Part model, mm, in its own coordinate system. A direction names the side the tool comes from. Round coordinates to 2 decimals unless told otherwise and drop trailing zeros. Loops run counter-clockwise (first coordinate to the right, second up) from the corner with the lowest first, then second, coordinate; pieces in that order, holes last. Notation, with made-up numbers: (33.25, 74) -> (59.25, 74) arc R15 cw to (59.25, 103) -> close; hole circle Ø10 at (86.25, 63.25). An arc over 180 degrees is marked (long way). Use a Markdown table: item, result. Add a question column.
Item 1: Cut at C-C, the plane y = 12. State how many separate pieces and enclosed holes the cut face has, plus the area to 3 significant figures.
Item 2: Which spindle directions (+Z, -Z, +X, -X, +Y, -Y) get a long thin tool onto all of the face, cutting with end or side? Do faces 1 (the face through (23, 6.35, 0)), 2 (the face through (30.8, 12.5, 25.1)), 3 (the face through (27.111, 18.942, -25.094)). Say none if no direction does.
Item 3: Two-plate mould, pull along X, no slides. Class faces 4 (the face through (-22.953, 39.572, 25.094)), 5 (the face through (5, 28, -25.4)), 6 (the face through (6.854, 38.289, -0.341)), 7 (the face through (-11, 6.35, 0)): pulls with the +X half, pulls with the -X half, needs draft (parallel to the pull), parting line crosses it, or undercut.
Item 4: Flat gauge pins, fed straight in: pin 1 (12 mm diameter, centred on x = -18.5, z = -2, fed in from +Y); pin 2 (3 mm diameter, centred on y = 31, z = -18, fed in from -X); pin 3 (12 mm diameter, centred on y = 14, z = -10, fed in from +X). Where does each tip first touch, or does it go through?
Item 5: Probe line 1 (X direction, y = 9.5, z = -14); line 2 (X direction, y = 11.5, z = -13); line 3 (Y direction, x = 17, z = -20). List the from-to ranges inside material, lowest first. Write a range as [from, to].
Item 6: Cut at B-B, the plane x = 19. List the corners of the cut face in (y, z), plus the area to 3 significant figures.
Autodesk Inventor part; units mm, degrees
ref_plane "YZ Plane" through (0, 0, 0) normal (1, 0, 0) x (0, 1, 0)
ref_plane "XZ Plane" through (0, 0, 0) normal (0, 1, 0) x (-1, 0, 0)
ref_plane "XY Plane" through (0, 0, 0) normal (0, 0, 1) x (1, 0, 0)
sketch "Sketch1" plane through (0, 0, 0) normal (0, 1, 0) x (-1, 0, 0)
  line L0 (-38.1, -25.4) -> (38.1, -25.4)
  line L1 (38.1, -25.4) -> (38.1, 25.4)
  line L2 (38.1, 25.4) -> (-38.1, 25.4)
  line L3 (-38.1, 25.4) -> (-38.1, -25.4)
  line L4 (-38.1, -25.4) -> (38.1, 25.4) construction
  line L5 (38.1, -25.4) -> (-38.1, 25.4) construction
  point P0 (0, 0)
  dimension "d0" = 76.2
  dimension "d1" = 50.8
extrude "Extrusion1" add sketch "Sketch1" along normal blind 6.35
sketch "Sketch2" plane through (38.1, 0, -25.4) normal (0, 0, -1) x (-1, 0, 0)
  line L0 (76.2, 6.35) -> (0, 6.35)
  line L1 (0, 6.35) -> (21.59, 6.35)
  line L2 (21.59, 6.35) -> (43.642, 79.2894)
  line L3 (76.2, 0) -> (76.2, 6.35)
  line L4 (43.642, 79.2894) -> (76.2, 6.35)
  line L5 (76.2, 6.35) -> (69.85, 6.35)
  line L6 (69.85, 6.35) -> (44.8636, 62.3267)
  line L7 (21.59, 6.35) -> (27.94, 6.35) construction
  line L8 (27.94, 6.35) -> (44.8636, 62.3267)
  line L9 (0, 6.35) -> (76.2, 6.35)
  line L10 (10.1092, 9.821) -> (9.0598, 6.35)
  line L11 (9.0598, 6.35) -> (5.2498, 6.35)
  line L12 (5.2498, 6.35) -> (9.0598, 19.7904)
  line L13 (9.0598, 19.7904) -> (12.64, 18.7755)
  line L14 (12.64, 18.7755) -> (9.9878, 9.4194)
  point P0 (38.1, 0)
  point P1 (5.2498, 6.35)
  point P2 (9.0598, 6.35)
  dimension "d4" = 21.59
  dimension "d5" = 76.2
  dimension "d6" = 6.35
  dimension "d7" = 6.35
  dimension "d9" = 11.4808
  dimension "d10" = 3.81
  dimension "d11" = 13.97
  dimension "d23" = 73.178
extrude "Extrusion2" add sketch "Sketch2" against normal up to surface (50.8 mm away) contours L0 L6 L8 L2 L4 | L0 L12 L13 L14 L10
sketch "Sketch3" plane through (0, 6.35, 0) normal (0, 1, 0) x (1, 0, 0)
  line L0 (32.8502, -25.4) -> (38.1, -25.4)
  line L1 (38.1, 25.4) -> (32.8502, 25.4)
  line L2 (32.8502, -25.4) -> (38.1, -25.4)
  line L3 (38.1, -25.4) -> (38.1, 25.4)
  line L4 (38.1, 25.4) -> (32.8502, 25.4)
  line L5 (32.8502, 25.4) -> (32.8502, -25.4)
  point P0 (0, 0)
extrude "Extrusion3" cut sketch "Sketch3" against normal blind 6.35
fillet "Fillet1" radius 1.016 1 edges at (32.8502, 6.35, 0)
fillet "Fillet2" radius 3.175 1 edges at (-5.542, 79.2894, 0)
fillet "Fillet3" radius 3.175 1 edges at (-38.1, 6.35, 0)
fillet "Fillet4" radius 1.016 10 edges at (-5.9152, 73.3838, -25.4) (-23.4195, 39.2385, -25.4) (-38.0303, 6.3352, -25.4) (-38.1, 2.8368, -25.4) (6.7168, 38.742, -25.4) (-5.9152, 73.3838, 25.4) (6.7168, 38.742, 25.4) (-38.0303, 6.3352, 25.4) (-38.1, 2.8368, 25.4) (-23.4195, 39.2385, 25.4)
fillet "Fillet5" radius 1.016 6 edges at (-10.795, 6.35, -25.4) (15.9793, 6.35, -25.4) (22.7751, 6.35, -25.4) (-10.795, 6.35, 25.4) (15.9793, 6.35, 25.4) (22.7751, 6.35, 25.4)
fillet "Fillet6" radius 1.016 4 edges at (27.2501, 19.283, -25.4) (27.2501, 19.283, 25.4) (29.0402, 19.7904, 0) (25.46, 18.7755, 0)
fillet "Fillet7" radius 1.016 8 edges at (32.8405, 6.3487, 25.4) (31.0645, 12.6494, 25.4) (28.8351, 19.423, 25.1024) (32.8502, 3.1044, 25.4) (32.8405, 6.3487, -25.4) (31.0645, 12.6494, -25.4) (28.8351, 19.423, -25.1024) (32.8502, 3.1044, -25.4)
equation "\"d12\" = d7"
properties part number "_3DPrint"
A:
| question | item | result |
|---|---|---|
| 1 | separate pieces | 3 |
| 1 | enclosed holes | 0 |
| 1 | area | 840 mm^2 |
| 2 | face 1 | +Z, -Z |
| 2 | face 2 | +Z, +X, +Y |
| 2 | face 3 | -Z, +Y |
| 3 | face 4 | pulls with the -X half |
| 3 | face 5 | needs draft |
| 3 | face 6 | undercut |
| 3 | face 7 | undercut |
| 4 | pin 1 | stops at y = 63.7 |
| 4 | pin 2 | stops at x = -27.77 |
| 4 | pin 3 | stops at x = 32.38 |
| 5 | line 1 | x = [-36.69, -30.34], [9.21, 15.56], [28.09, 31.96] |
| 5 | line 2 | x = [-35.8, -29.45], [8.6, 14.95], [27.52, 31.39] |
| 5 | line 3 | y = [0, 6.35] |
| 6 | outline | (0, -25.4) -> (5.33, -25.4) arc R1.02 ccw to (6.35, -24.38) -> (6.35, 24.38) arc R1.02 ccw to (5.33, 25.4) -> (0, 25.4) -> close |
| 6 | area | 322 mm^2 |
